from build123d import *

# Parameters (mm, degrees)
SKETCH_1_R          = 42
EXTRUDE_1_DEPTH     = 20
EXTRUDE_2_DEPTH     = 5
SKETCH_4_R          = 42
CUT_EXTRUDE_1_DEPTH = 15


with BuildPart() as part:
    # Sketch 1 → Extrude 1 (new body)
    with BuildSketch(Plane.XY):
        Circle(SKETCH_1_R)
    extrude(amount=EXTRUDE_1_DEPTH)



with BuildPart() as body_2:
    # Sketch 2 → Revolve 1 (revolve)
    with BuildSketch(Plane.XY.offset(20), mode=Mode.PRIVATE) as revolve_1_sk:
        with BuildLine():
            Line((100, 20), (100, 15))
            ThreePointArc((100, 15), (86.583592135, 6.708203932), (88, -9))
            Line((88, -9), (80, -9))
            Line((80, -9), (80, 20))
            Line((80, 20), (100, 20))
        make_face()
    revolve(revolve_1_sk.sketch.rotate(Axis((100, 22.717290725, 20), (0, -1, 0)), 270), axis=Axis((100, 22.717290725, 20), (0, -1, 0)))


with BuildPart() as part_1:
    add(part.part)

    add(body_2.part)  # Extrude 2 merges body 2
    # Sketch 3 → Extrude 2 (add, symmetric)
    with BuildSketch(Plane.XY.offset(20)):
        with BuildLine():
            Line((14.069453744, 39.573355574), (86, 14))
            Line((86, 14), (86, -3))
            Line((86, -3), (19.208719722, -37.350034627))
            ThreePointArc((19.208719722, -37.350034627), (-41.906577017, -2.79978619), (14.069453744, 39.573355574))
        make_face()
    extrude(amount=EXTRUDE_2_DEPTH, both=True)

    # Sketch 4 → Cut-Extrude 1 (cut)
    with BuildSketch(Plane(origin=(0, 0, 0), x_dir=(-1, 0, 0), z_dir=(0, 0, -1))):
        Circle(SKETCH_4_R)
    extrude(amount=-CUT_EXTRUDE_1_DEPTH, mode=Mode.SUBTRACT)


solid = part_1.part
Input: part model. Units: mm. Frame: model coordinates. A direction names the side the tool comes from. Round coordinates to 2 decimals unless told otherwise and drop trailing zeros. Loops run counter-clockwise (first coordinate to the right, second up) from the corner with the lowest first, then second, coordinate; pieces in that order, holes last. Notation, with made-up numbers: (13.5, 14) -> (59.5, 14) arc R14 ccw to (59.5, 22) -> close; hole circle Ø11 at (-34.75, 54.5). An arc over 180 degrees is marked (long way). Answer as a JSON object with one key per item and string values. Group by question number.
1) Draft query along Z for faces 1 (the flat face through (86, 1, 20)), 2 (the flat face through (50.352, -21.333, 20.07)), 3 (the flat face through (20, 1, 15)). Return one class per face: +Z half, -Z half, draft (parallel to the pull), parting line (faces both ways), or undercut.
2) Ray query, L1, parallel to Z at x = 55.5, y = 3.5; L2, parallel to X at y = -2.5, z = 32; L3, parallel to Z at x = 105.5, y = -5.5. Return the intervals inside material, ascending.
3) Pin query (flat end, axial travel): pin 1 (12 mm diameter, centred on x = 109, z = 17, fed in from -Y); pin 2 (5 mm diameter, centred on x = -16.5, y = -14, fed in from -Z); pin 3 (1 mm diameter, centred on y = 14, z = 34, fed in from -X); pin 4 (12 mm diameter, centred on y = 30.5, z = 5, fed in from -X). Return the tip coordinate at first contact, or that it passes through.
4) Section query D-D on x = 100. Output: boundary loops of the cut face in (y, z), plus the area to 3 significant figures.
5) Section query B-B on x = 0. Output: boundary loops of the cut face in (y, z), plus the area to 3 significant figures.
6) Section query C-C on z = 33.5. Output: boundary loops of the cut face in (x, y), plus the area to 3 significant figures.
7) Section query A-A on y = 0. Output: boundary loops of the cut face in (x, z), plus the area to 3 significant figures.
8) Reachability of faces 4 (the flat face through (109, -9, 11)), 5 (the flat face through (20, 1, 25)), 6 (the flat face through (100, 20, 20)) from +Z, -Z, +X, -X, +Y, -Y: full face, straight path, thin tool, end or side. Return the list, or none.
Reply:
{
 "1": {"face 1": "undercut", "face 2": "draft", "face 3": "-Z half"},
 "2": {"L1": "z = 15 to 25", "L2": "x = 84 to 91.35, 108.65 to 116", "L3": "z = 0.77 to 7.17, 32.83 to 39.23"},
 "3": {"pin 1": "stops at y = -9", "pin 2": "stops at z = 15", "pin 3": "stops at x = 85.24", "pin 4": "passes through"},
 "4": {"outline": "(-9, 0) -> (20, 0) -> (20, 40) -> (-9, 40) -> (-9, 32) arc R15 cw (long way) to (-9, 8) -> close", "area": "554 mm2"},
 "5": {"outline": "(-42, 15) -> (42, 15) -> (42, 25) -> (-42, 25) -> close", "area": "840 mm2"},
 "6": {"outline": "(85.24, -9) -> (114.76, -9) -> (114.76, 20) -> (85.24, 20) -> close; hole circle Ø13.08 at (100, 0)", "area": "722 mm2"},
 "7": {"outline": "(-42, 15) -> (80.64, 15) arc R20 ccw (long way) to (80.64, 25) -> (-42, 25) -> close; hole (85.86, 15) arc R15 ccw (long way) to (85.86, 25) -> (86, 25) -> (86, 15) -> close", "area": "1,780 mm2"},
 "8": {"face 4": "+Z, -Z, +X, -Y", "face 5": "+Z, -X, +Y, -Y", "face 6": "+Z, -Z, +X, +Y"}
}
